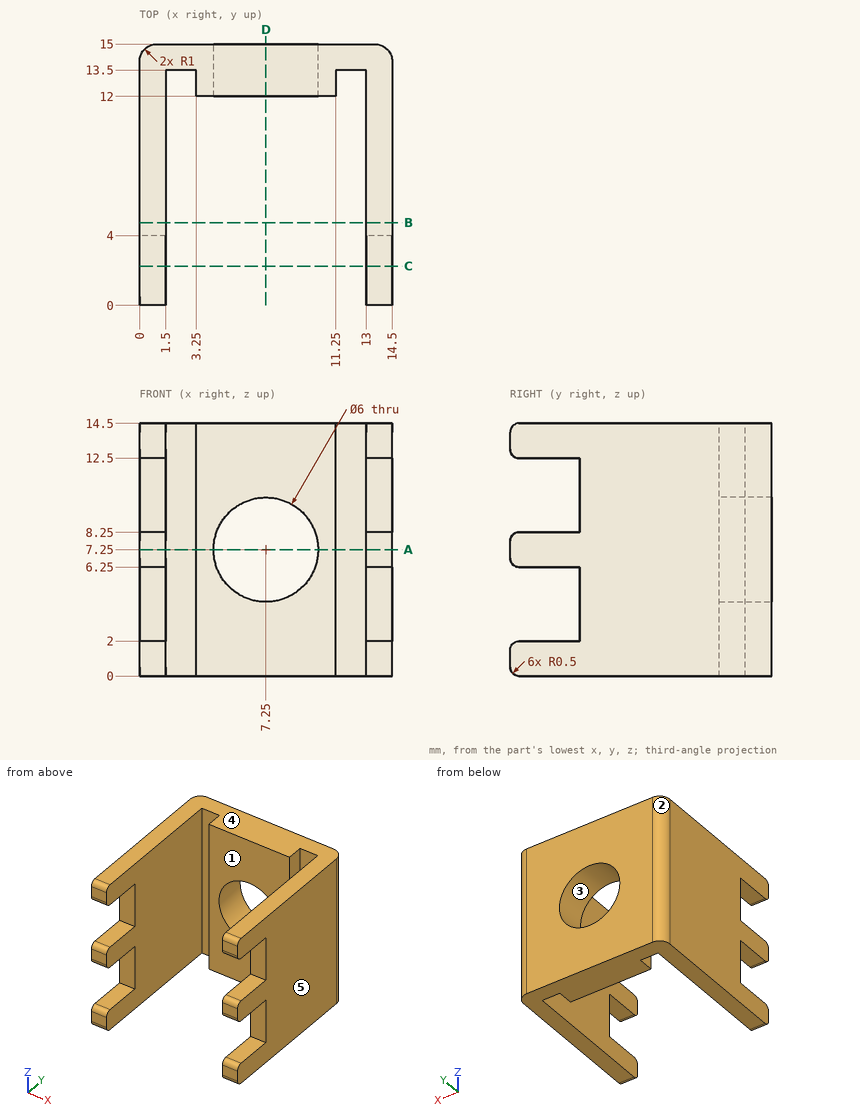
Verification items for this drawing (mm, ordinates from the low corner). A direction names the side the tool comes from. Round coordinates to 2 decimals unless told otherwise and drop trailing zeros. Order: outer loops, then holes, each group sorted by start corner. A loop starts at its lowest first (then second) coordinate and runs counter-clockwise, first axis right, second up. Notation, with made-up numbers: M -39.5,67.25 L -3.5,67.25 A20 ccw -3.5,90.25 Z; hole C 86,-39.75 d5. An arc over 180 degrees is marked long. Answer in a Markdown table with one row per item. Add a question column.
Item 1: Sectioned sample at D-D, the plane x = 7.25. Enter the section's corners in (y, z).
Item 2: Sectioned sample at B-B, the plane y = 4.75. Enter the section's corners in (x, z).
Item 3: Draft check along Z on the marked faces 3, 4 and 5. Enter one of: released by +Z, released by -Z, zero draft, split by the parting line, or undercut.
Item 4: Sectioned sample at C-C, the plane y = 2.25. Enter the section's corners in (x, z), plus the area to 3 significant figures.
Item 5: Set-up check for the marked faces 1 and 2: record each of +Z, -Z, +X, -X, +Y, -Y from which the full face is reachable in a straight line by a thin tool's end or side.
Item 6: Material ranges on L1, parallel to X at y = 12.8, z = 7.25; L2, parallel to X at y = 11, z = 7; L3, parallel to X at y = 14.05, z = 7.25, recorded low to high. Write a range as [from, to].
Item 7: Depth check by flat-ended pin: pin 1 Ø4 at (x, z) = (6, 3.5) entering from -Y; pin 2 Ø0.8 at (x, z) = (1, 3) entering from -Y; pin 3 Ø3.5 at (x, z) = (7.25, 7.25) entering from +Y. Enter the tip coordinate at first touch or a pass-through.
Item 8: Sectioned sample at A-A, the plane z = 7.25. Enter the section's corners in (x, y), plus the area to 3 significant figures.
Filled in:
| question | item | result |
|---|---|---|
| 1 | outline | M 12,0 L 15,0 L 15,4.25 L 12,4.25 Z; M 12,10.25 L 15,10.25 L 15,14.5 L 12,14.5 Z |
| 2 | outline | M 0,0 L 1.5,0 L 1.5,14.5 L 0,14.5 Z; M 13,0 L 14.5,0 L 14.5,14.5 L 13,14.5 Z |
| 3 | face 3 | undercut |
| 3 | face 4 | released by +Z |
| 3 | face 5 | zero draft |
| 4 | outline | M 0,0 L 1.5,0 L 1.5,2 L 0,2 Z; M 0,6.25 L 1.5,6.25 L 1.5,8.25 L 0,8.25 Z; M 0,12.5 L 1.5,12.5 L 1.5,14.5 L 0,14.5 Z; M 13,0 L 14.5,0 L 14.5,2 L 13,2 Z; M 13,6.25 L 14.5,6.25 L 14.5,8.25 L 13,8.25 Z; M 13,12.5 L 14.5,12.5 L 14.5,14.5 L 13,14.5 Z |
| 4 | area | 18.0 mm² |
| 5 | face 1 | +Z, -Z, -Y |
| 5 | face 2 | +Z, -Z, -X, +Y |
| 6 | L1 | x = [0, 1.5], [3.25, 4.25], [10.25, 11.25], [13, 14.5] |
| 6 | L2 | x = [0, 1.5], [13, 14.5] |
| 6 | L3 | x = [0, 4.25], [10.25, 14.5] |
| 7 | pin 1 | stops at y = 12 |
| 7 | pin 2 | stops at y = 4 |
| 7 | pin 3 | passes through |
| 8 | outline | M 0,0 L 1.5,0 L 1.5,13.5 L 3.25,13.5 L 3.25,12 L 4.25,12 L 4.25,15 L 1,15 A1 ccw 0,14 Z; M 10.25,12 L 11.25,12 L 11.25,13.5 L 13,13.5 L 13,0 L 14.5,0 L 14.5,14 A1 ccw 13.5,15 L 10.25,15 Z |
| 8 | area | 55.8 mm² |
